For this review, take the finished solid that the model builds, in its own axes (mm). A direction names the side the tool comes from. Round coordinates to 2 decimals unless told otherwise and drop trailing zeros. Order: outer loops, then holes, each group sorted by start corner. A loop starts at its lowest first (then second) coordinate and runs counter-clockwise, first axis right, second up. Notation, with made-up numbers: M 63.5,25 L 114.5,25 A12 cw 114.5,29 Z; hole C 58,-15.75 d6. An arc over 180 degrees is marked long. Put each result on its own line as item: value.
from build123d import *

# Parameters (mm, degrees)
F0_R     = 3.175
F0_W     = 19.05
F0_H     = 15.24
F1_DEPTH = 17.78


with BuildPart() as f1:
    # F0 (on Front) → F1 (new body)
    with BuildSketch(Plane.XZ):
        with BuildLine():
            Line((12.07617, 59.472699), (12.07617, 58.202699))
            Line((12.07617, 58.202699), (12.07617, 42.327699))
            Line((12.07617, 42.327699), (12.07617, 26.452699))
            Line((12.07617, 26.452699), (12.07617, 25.182699))
            ThreePointArc((12.07617, 25.182699), (14.494003, 19.345532), (20.33117, 16.927699))
            Line((20.33117, 16.927699), (50.17617, 16.927699))
            Line((50.17617, 16.927699), (50.17617, 23.277699))
            Line((50.17617, 23.277699), (56.52617, 23.277699))
            Line((56.52617, 23.277699), (56.52617, 16.927699))
            Line((56.52617, 16.927699), (64.736042, 16.927699))
            Line((64.736042, 16.927699), (69.22617, 21.417827))
            Line((69.22617, 21.417827), (69.22617, 63.237571))
            Line((69.22617, 63.237571), (64.736042, 67.727699))
            Line((64.736042, 67.727699), (20.33117, 67.727699))
            ThreePointArc((20.33117, 67.727699), (14.494003, 65.309865), (12.07617, 59.472699))
        make_face()
        with Locations((24.77617, 26.452699)):
            Circle(F0_R, mode=Mode.SUBTRACT)
        with Locations((43.82617, 41.057699)):
            Rectangle(F0_W, F0_H, mode=Mode.SUBTRACT)
        with Locations((24.77617, 58.202699)):
            Circle(F0_R, mode=Mode.SUBTRACT)
    extrude(amount=F1_DEPTH)


solid = f1.part
(1) Draft analysis for pull direction Z (two halves, no side actions). For faces 4 (the face through (12.076, -9, 43)), 5 (the face through (44, -9, 48.678)), 6 (the face through (66.95, -8.77, 19.14)), state which applies: released by +Z, released by -Z, zero draft, split by the parting line, or undercut.
A:
face 4: zero draft
face 5: undercut
face 6: released by -Z
(2) Add section D-D on x = 25.5. Give the boundary of the cut face in (y, z).
A:
outline: M -17.78,16.93 L 0,16.93 L 0,23.36 L -17.78,23.36 Z; M -17.78,29.54 L 0,29.54 L 0,55.11 L -17.78,55.11 Z; M -17.78,61.29 L 0,61.29 L 0,67.73 L -17.78,67.73 Z
(3) Insertion check: pin 1 Ø7 at (x, y) = (54, -7.5) entering from -Z; pin 2 Ø3 at (y, z) = (-7, 21) entering from -X. Each pin has a flat end and moves straight along its axis. Give the tip position at first contact, or say it passes through.
A:
pin 1: stops at z = 16.93
pin 2: stops at x = 12.52
(4) To check wall thickness, follow L1, parallel to X at y = -9.5, z = 44.5; L2, parallel to Z at x = 47, y = -1.5; L3, parallel to Z at x = 24.5, y = -11. State the ranges of each line that lie inside material, in increasing order.
A:
L1: x = 12.08 to 34.3, 53.35 to 69.23
L2: z = 16.93 to 33.44, 48.68 to 67.73
L3: z = 16.93 to 23.29, 29.62 to 55.04, 61.37 to 67.73
(5) Add section B-B on z = 48. Give the boundary of the cut face in (x, y), then the cut area to 3 significant figures.
A:
outline: M 12.08,-17.78 L 34.3,-17.78 L 34.3,0 L 12.08,0 Z; M 53.35,-17.78 L 69.23,-17.78 L 69.23,0 L 53.35,0 Z
area: 677 mm2
(6) For faces 1 (the face through (53.351, -9, 41)), 2 (the face through (50.176, -9, 20)), 3 (the face through (43, -9, 67.728)), list the 3-axis set-ups (+Z, -Z, +X, -X, +Y, -Y) from which the entire face can be reached by the end or side of a thin tool; tool diameter is ignored.
A:
face 1: +Y, -Y
face 2: -Z, +Y, -Y
face 3: +Z, +X, -X, +Y, -Y
(7) Add section A-A on x = 44. Give the boundary of the cut face in (y, z).
A:
outline: M -17.78,16.93 L 0,16.93 L 0,33.44 L -17.78,33.44 Z; M -17.78,48.68 L 0,48.68 L 0,67.73 L -17.78,67.73 Z
(8) Add section C-C on y = -10.25. Give the boundary of the cut face in (x, z) (3 decimals).
A:
outline: M 12.076,25.183 A8.255 ccw 20.331,16.928 L 50.176,16.928 L 50.176,23.278 L 56.526,23.278 L 56.526,16.928 L 64.736,16.928 L 69.226,21.418 L 69.226,63.238 L 64.736,67.728 L 20.331,67.728 A8.255 ccw 12.076,59.473 Z; hole C 24.776,26.453 d6.35; hole C 24.776,58.203 d6.35; hole M 34.301,33.438 L 53.351,33.438 L 53.351,48.678 L 34.301,48.678 Z
